from build123d import *

# Parameters (mm, degrees)
SKETCH1_W           = 95.25
SKETCH1_H           = 76.2
BOSS_EXTRUDE1_DEPTH = 2.794
SKETCH2_R           = 1.8288
CUT_EXTRUDE1_DEPTH  = 62.053722745
SKETCH3_R           = 1.524
CUT_EXTRUDE2_DEPTH  = 62.053722745


with BuildPart() as part:
    # Sketch1 → Boss-Extrude1 (new body)
    with BuildSketch(Plane(origin=(0, 0, 0), x_dir=(1, 0, 0), z_dir=(0, 1, 0))):
        Rectangle(SKETCH1_W, SKETCH1_H)
    extrude(amount=BOSS_EXTRUDE1_DEPTH)

    # Sketch2 → Cut-Extrude1 (cut, through all)
    with BuildSketch(Plane(origin=(0, 2.794, 0), x_dir=(1, 0, 0), z_dir=(0, 1, 0))):
        with Locations(Location((-38.1, 31.75, 0), (0, 0, 270))):
            Circle(SKETCH2_R)
        with Locations(Location((-19.05, 31.75, 0), (0, 0, 270))):
            Circle(SKETCH2_R)
        with Locations(Location((0, 31.75, 0), (0, 0, 270))):
            Circle(SKETCH2_R)
        with Locations(Location((19.05, 31.75, 0), (0, 0, 270))):
            Circle(SKETCH2_R)
        with Locations(Location((38.1, 31.75, 0), (0, 0, 270))):
            Circle(SKETCH2_R)
    extrude(amount=-CUT_EXTRUDE1_DEPTH, mode=Mode.SUBTRACT)

    # Sketch3 → Cut-Extrude2 (cut, through all)
    with BuildSketch(Plane(origin=(0, 2.794, 0), x_dir=(1, 0, 0), z_dir=(0, 1, 0))):
        with Locations(Location((-12.7, 12.7, 0), (0, 0, 270))):
            Circle(SKETCH3_R)
        with Locations(Location((12.7, 12.7, 0), (0, 0, 270))):
            Circle(SKETCH3_R)
    extrude(amount=-CUT_EXTRUDE2_DEPTH, mode=Mode.SUBTRACT)


solid = part.part
Verification items for the finished model (mm, model axes). Round coordinates to 2 decimals unless told otherwise and drop trailing zeros. Order: outer loops, then holes, each group sorted by start corner. A loop starts at its lowest first (then second) coordinate and runs counter-clockwise, first axis right, second up. Notation, with made-up numbers: (48, 23.5) -> (73, 23.5) arc R19 cw to (73, 43.5) -> close; hole circle Ø8 at (-18.75, 5). An arc over 180 degrees is marked (long way). Put each result on its own line as item: value.
1) Section check C-C (x = 19.05). Record the cut outline in (y, z), then the cut area to 3 significant figures.
Final values:
outline: (0, -38.1) -> (2.79, -38.1) -> (2.79, -33.58) -> (0, -33.58) -> close; (0, -29.92) -> (2.79, -29.92) -> (2.79, 38.1) -> (0, 38.1) -> close
area: 203 mm^2
2) Section check A-A (z = -31.75). Record the cut outline in (x, y) (3 decimals), then the cut area to 3 significant figures.
Final values:
outline: (-47.625, 0) -> (-39.929, 0) -> (-39.929, 2.794) -> (-47.625, 2.794) -> close; (-36.271, 0) -> (-20.879, 0) -> (-20.879, 2.794) -> (-36.271, 2.794) -> close; (-17.221, 0) -> (-1.829, 0) -> (-1.829, 2.794) -> (-17.221, 2.794) -> close; (1.829, 0) -> (17.221, 0) -> (17.221, 2.794) -> (1.829, 2.794) -> close; (20.879, 0) -> (36.271, 0) -> (36.271, 2.794) -> (20.879, 2.794) -> close; (39.929, 0) -> (47.625, 0) -> (47.625, 2.794) -> (39.929, 2.794) -> close
area: 215 mm^2
3) Section check B-B (x = -12.7). Record the cut outline in (y, z).
Final values:
outline: (0, -38.1) -> (2.79, -38.1) -> (2.79, -14.22) -> (0, -14.22) -> close; (0, -11.18) -> (2.79, -11.18) -> (2.79, 38.1) -> (0, 38.1) -> close
4) Material ranges on line 1 (X direction, y = 1.15, z = -31.75) (3 decimals); line 2 (X direction, y = 1.9, z = -13) (3 decimals); line 3 (Z direction, x = -12.5, y = 1.1), recorded low to high.
Final values:
line 1: x = -47.625 to -39.929, -36.271 to -20.879, -17.221 to -1.829, 1.829 to 17.221, 20.879 to 36.271, 39.929 to 47.625
line 2: x = -47.625 to -14.194, -11.206 to 11.206, 14.194 to 47.625
line 3: z = -38.1 to -14.21, -11.19 to 38.1
5) Depth check by flat-ended pin: pin 1 (8 mm diameter, centred on x = 36, z = 18, fed in from -Y); pin 2 (2.5 mm diameter, centred on x = 12.7, z = -12.7, fed in from -Y). Enter the tip coordinate at first touch or a pass-through.
Final values:
pin 1: stops at y = 0
pin 2: passes through
6) Mould release check, pull along Z, two halves, no side actions. Record for faces 1 (the flat face through (-1, 0, -1)), 2 (the cylindrical face through (-12.633, 1.417, -14.223)), 3 (the cylindrical face through (-20.672, 1.417, -30.906)), 4 (the flat face through (-1, 1, -38.1)): +Z half, -Z half, draft (parallel to the pull), parting line (faces both ways), or undercut.
Final values:
face 1: draft
face 2: undercut
face 3: undercut
face 4: -Z half
